Answer from the drawing. Dimensions are ordinates in mm from the lowest x, y and z of the part. Give positions to 0.01 mm unless a question says otherwise; leave off trailing zeros. Order: outer loops, then holes, each group sorted by start corner. A loop starts at its lowest first (then second) coordinate and runs counter-clockwise, first axis right, second up.
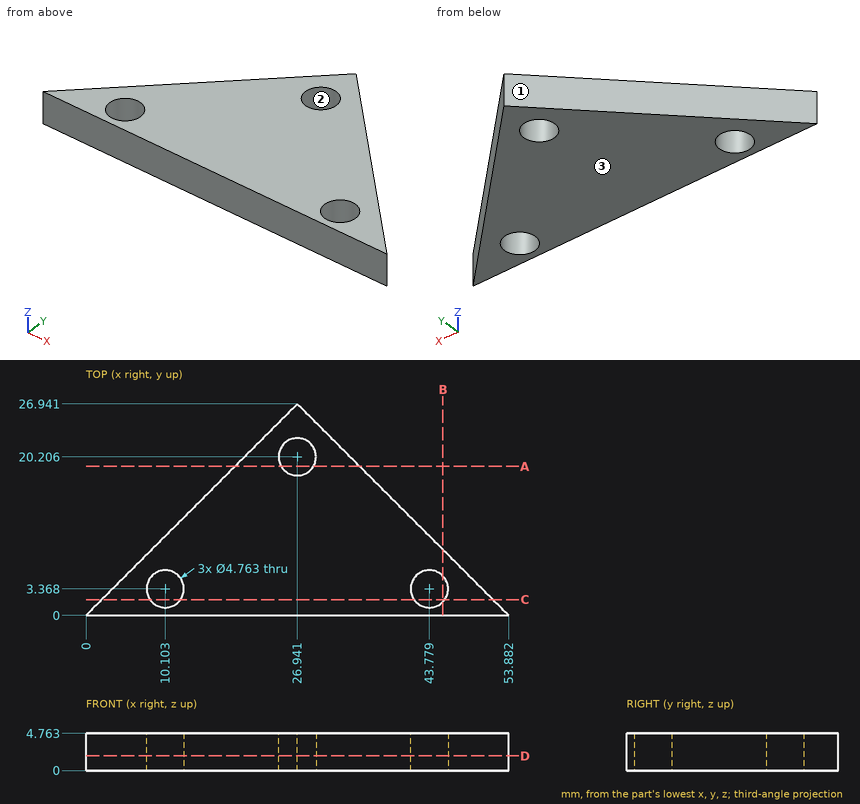
1) The part is cut by section A-A on y = 19. Determine the outline of the cut face in (x, z) (1 decimal).
Final values:
outline: (19, 0) - (24.9, 0) - (24.9, 4.8) - (19, 4.8) - close; (29, 0) - (34.9, 0) - (34.9, 4.8) - (29, 4.8) - close
2) The part is cut by section D-D on z = 1.9. Determine the outline of the cut face in (x, y) (1 decimal).
Final values:
outline: (0, 0) - (53.9, 0) - (26.9, 26.9) - close; hole circle Ø4.8 at (10.1, 3.4); hole circle Ø4.8 at (26.9, 20.2); hole circle Ø4.8 at (43.8, 3.4)
3) For a pull along X with two mould halves and no side action, classify the marked faces 1, 2 and 3 as released by +X, released by -X, zero draft, split by the parting line, or undercut.
Final values:
face 1: released by -X
face 2: undercut
face 3: zero draft
4) Given pin 1 (2 mm diameter, centred on y = 9.5, z = 2, fed in from -X); pin 2 (1 mm diameter, centred on y = 21, z = 3, fed in from +X), each flat-ended and moving along its own axis, determine where each tip first touches the part or whether it passes through.
Final values:
pin 1: stops at x = 8.5
pin 2: stops at x = 33.38
5) The part is cut by section C-C on y = 2. Determine the outline of the cut face in (x, z).
Final values:
outline: (2, 0) - (8.15, 0) - (8.15, 4.76) - (2, 4.76) - close; (12.05, 0) - (41.83, 0) - (41.83, 4.76) - (12.05, 4.76) - close; (45.73, 0) - (51.88, 0) - (51.88, 4.76) - (45.73, 4.76) - close
6) The part is cut by section B-B on x = 45.5. Determine the outline of the cut face in (y, z).
Final values:
outline: (0, 0) - (1.72, 0) - (1.72, 4.76) - (0, 4.76) - close; (5.01, 0) - (8.38, 0) - (8.38, 4.76) - (5.01, 4.76) - close
7) Consider L1, parallel to X at y = 21.5, z = 2.25 (1 decimal); L2, parallel to X at y = 5.5, z = 1.6 (1 decimal); L3, parallel to X at y = 18.5, z = 2.7 (1 decimal). Determine where each line is inside the solid, lowest interval first.
Final values:
L1: x = 21.5 to 24.9, 28.9 to 32.4
L2: x = 5.5 to 9, 11.2 to 42.7, 44.8 to 48.4
L3: x = 18.5 to 25.3, 28.6 to 35.4
